```python
from build123d import *

# Parameters (mm, degrees)
F0_W      = 74
F0_H      = 32
F1_DEPTH  = 3
F2_W      = 74
F2_H      = 2
F3_DEPTH  = 60
F4_W      = 74
F4_H      = 32
F5_DEPTH  = 3
F6_W      = 9
F6_H      = 1.5
F7_DEPTH  = 5
F8_W      = 9
F8_H      = 1.5
F9_DEPTH  = 5
F11_DEPTH = 66


with BuildPart() as f1:
    # F0 (on Top) → F1 (new body)
    with BuildSketch(Plane.XY):
        Rectangle(F0_W, F0_H)
    extrude(amount=F1_DEPTH)

    # F2 (on face) → F3 (join)
    with BuildSketch(Plane(origin=(0, 0, 0), x_dir=(1, 0, 0), z_dir=(0, 0, -1))):
        with Locations((0, 15)):
            Rectangle(F2_W, F2_H)
    extrude(amount=F3_DEPTH)

    # F4 (on face) → F5 (join)
    with BuildSketch(Plane(origin=(0, 0, -60), x_dir=(1, 0, 0), z_dir=(0, 0, -1))):
        Rectangle(F4_W, F4_H)
    extrude(amount=F5_DEPTH)

    # F6 (on face) → F7 (join)
    with BuildSketch(Plane(origin=(0, 16, 0), x_dir=(-1, 0, 0), z_dir=(0, 1, 0))):
        with Locations((0, 1.5)):
            Rectangle(F6_W, F6_H)
    extrude(amount=F7_DEPTH)

    # F8 (on face) → F9 (join)
    with BuildSketch(Plane(origin=(0, 16, 0), x_dir=(-1, 0, 0), z_dir=(0, 1, 0))):
        with Locations((0, -61.5)):
            Rectangle(F8_W, F8_H)
    extrude(amount=F9_DEPTH)

    # F10 (on face) → F11 (cut, through all)
    with BuildSketch(Plane.XY.offset(3)):
        with BuildLine():
            Line((12.5, 16), (12.5, 3))
            ThreePointArc((12.5, 3), (19, -3.5), (25.5, 3))
            Line((25.5, 3), (25.5, 16))
            Line((25.5, 16), (12.5, 16))
        make_face()
    extrude(amount=-F11_DEPTH, mode=Mode.SUBTRACT)


solid = f1.part
```
For this review, take the finished solid that the model builds, in its own axes (mm). A direction names the side the tool comes from. Coordinates: 2 decimals unless noted, no trailing zeros. Write each loop counter-clockwise with the first axis right and the second up, starting at its lowest first coordinate (ties: lowest second). Pieces come first, ordered by that corner, then holes. Notation, with made-up numbers: (30, 75.25) - (56, 75.25) arc R25 ccw to (56, 95.25) - close; hole circle Ø6 at (28.5, 22.25). An arc over 180 degrees is marked (long way). Answer in a Markdown table with one row per item. Add a question column.
Q1. For P1, Ø5, axis at x = 8.5, z = -43, coming from the +Y side; P2, Ø0.8, axis at y = 18.5, z = 1.5, coming from the -X side; P3, Ø1.5, axis at x = 30.5, z = 1.5, coming from the +Y side; P4, Ø8, axis at y = 17, z = -54, coming from the +X side, all flat-tipped, find the tip position at first contact; note any pin that passes through.
Q2. We need section D-D, the plane y = 18.5. State the section outline as (x, z) points, and give its area (3 significant figures).
Q3. We need section B-B, the plane y = -5. State the section outline as (x, z) points, and give its area (3 significant figures).
Q4. For probe 1 along Z at (x, y) = (7, -5.5); probe 2 along Y at (x, z) = (-10.5, -54), list the stretches that pass through material, from the lowest coordinate up.
Q5. We need section A-A, the plane y = 4. State the section outline as (x, z) points, and give its area (3 significant figures).
Q6. Draft analysis for pull direction X (two halves, no side actions). For faces 1 (the flat face through (25.5, 9, 2)), 2 (the flat face through (12.5, 10, -61)), 3 (the flat face through (0, 18, -60.75)), 4 (the flat face through (37, -14.15, -29.85)), state which applies: +X half, -X half, draft (parallel to the pull), parting line (faces both ways), or undercut.
Q7. Tool access review of faces 5 (the flat face through (0, 18, 2.25)), 6 (the flat face through (31, 16, 1)), 7 (the flat face through (-1, 1, -60)), 8 (the flat face through (-1, 0, -63)), 9 (the flat face through (25.5, 9, -61)): name each direction out of +Z, -Z, +X, -X, +Y, -Y from which nothing blocks a thin tool from reaching the whole face with its end or side.
Q8. We need section C-C, the plane x = 19. State the section outline as (y, z) points.
Answer list:
| question | item | result |
|---|---|---|
| 1 | P1 | stops at y = -14 |
| 1 | P2 | stops at x = -4.5 |
| 1 | P3 | stops at y = 16 |
| 1 | P4 | passes through |
| 2 | outline | (-4.5, -62.25) - (4.5, -62.25) - (4.5, -60.75) - (-4.5, -60.75) - close; (-4.5, 0.75) - (4.5, 0.75) - (4.5, 2.25) - (-4.5, 2.25) - close |
| 2 | area | 27.0 mm2 |
| 3 | outline | (-37, -63) - (37, -63) - (37, -60) - (-37, -60) - close; (-37, 0) - (37, 0) - (37, 3) - (-37, 3) - close |
| 3 | area | 444 mm2 |
| 4 | probe 1 | z = -63 to -60, 0 to 3 |
| 4 | probe 2 | y = -16 to -14 |
| 5 | outline | (-37, -63) - (12.5, -63) - (12.5, -60) - (-37, -60) - close; (-37, 0) - (12.5, 0) - (12.5, 3) - (-37, 3) - close; (25.5, -63) - (37, -63) - (37, -60) - (25.5, -60) - close; (25.5, 0) - (37, 0) - (37, 3) - (25.5, 3) - close |
| 5 | area | 366 mm2 |
| 6 | face 1 | undercut |
| 6 | face 2 | undercut |
| 6 | face 3 | draft |
| 6 | face 4 | +X half |
| 7 | face 5 | +Z, +X, -X, +Y |
| 7 | face 6 | +Z, -Z, +X, +Y |
| 7 | face 7 | +X, -X, +Y |
| 7 | face 8 | -Z, +X, -X, +Y, -Y |
| 7 | face 9 | +Z, -Z, +Y |
| 8 | outline | (-16, -63) - (-3.5, -63) - (-3.5, -60) - (-14, -60) - (-14, 0) - (-3.5, 0) - (-3.5, 3) - (-16, 3) - close |
